from build123d import *

# Parameters (mm, degrees)
SKETCH_1_W          = 4.39
SKETCH_1_H          = 6.1
EXTRUDE_1_DEPTH     = 4.65
SKETCH_2_W          = 1
SKETCH_2_H          = 3
CUT_EXTRUDE_1_DEPTH = 0.01
SKETCH_3_R          = 0.25
EXTRUDE_2_DEPTH     = 3


with BuildPart() as part:
    # Эскиз1 → Бобышка-Вытянуть1 (new body)
    with BuildSketch(Plane.XY):
        with Locations((2.195, 3.05)):
            Rectangle(SKETCH_1_W, SKETCH_1_H)
    extrude(amount=EXTRUDE_1_DEPTH)

    # Эскиз2 → Вырез-Вытянуть1 (cut)
    with BuildSketch(Plane.XY.offset(4.65)):
        with Locations((1.1, 3.05)):
            Rectangle(SKETCH_2_W, SKETCH_2_H)
        with Locations((3.29, 3.05)):
            Rectangle(SKETCH_2_W, SKETCH_2_H)
    extrude(amount=-CUT_EXTRUDE_1_DEPTH, mode=Mode.SUBTRACT)

    # Эскиз3 → Бобышка-Вытянуть2 (add)
    with BuildSketch(Plane.XY):
        with Locations((1.14, 1.78)):
            Circle(SKETCH_3_R)
        with Locations((3.25, 1.78)):
            Circle(SKETCH_3_R)
        with Locations((3.25, 4.32)):
            Circle(SKETCH_3_R)
        with Locations((1.14, 4.32)):
            Circle(SKETCH_3_R)
    extrude(amount=-EXTRUDE_2_DEPTH)


solid = part.part
Design review of the part built by this model. Coordinates are the model's own, in mm. A direction names the side the tool comes from. Round coordinates to 2 decimals unless told otherwise and drop trailing zeros. Loops run counter-clockwise (first coordinate to the right, second up) from the corner with the lowest first, then second, coordinate; pieces in that order, holes last. Notation, with made-up numbers: (2, 2) - (33, 2) arc R16 ccw to (33, 30) - close; hole circle Ø4 at (45.5, 82.5). An arc over 180 degrees is marked (long way). One line per item, written item: value. Start each with the question number.
1) Insertion check: pin 1 Ø1.3 at (x, y) = (1.5, 4) entering from -Z; pin 2 Ø2 at (x, z) = (3, -1.5) entering from +Y. Each pin has a flat end and moves straight along its axis. Give the tip position at first contact, or say it passes through.
2) To check wall thickness, follow L1, parallel to Z at x = 2.55, y = 3.5; L2, parallel to Y at x = 3.3, z = -0.75. State the ranges of each line that lie inside material, in increasing order. Write a range as from..to.
3) Consider section A-A on z = -2. Give the boundary of the cut face in (x, y).
4) For faces 1 (the flat face through (1, 3, 4.64)), 2 (the flat face through (2, 3, 0)), 3 (the flat face through (2, 3, 4.65)), list the 3-axis set-ups (+Z, -Z, +X, -X, +Y, -Y) from which the entire face can be reached by the end or side of a thin tool; tool diameter is ignored.
5) Draft analysis for pull direction X (two halves, no side actions). For faces 4 (the flat face through (3, 3, 4.64)), 5 (the flat face through (2, 0, 2)), 6 (the flat face through (4.39, 3, 2)), state which applies: +X half, -X half, draft (parallel to the pull), parting line (faces both ways), or undercut.
Reported:
1. pin 1: stops at z = -3
1. pin 2: stops at y = 4.57
2. L1: z = 0..4.65
2. L2: y = 1.54..2.02, 4.08..4.56
3. outline: circle Ø0.5 at (1.14, 1.78); circle Ø0.5 at (1.14, 4.32); circle Ø0.5 at (3.25, 1.78); circle Ø0.5 at (3.25, 4.32)
4. face 1: +Z
4. face 2: -Z
4. face 3: +Z, +X, -X, +Y, -Y
5. face 4: undercut
5. face 5: draft
5. face 6: +X half
